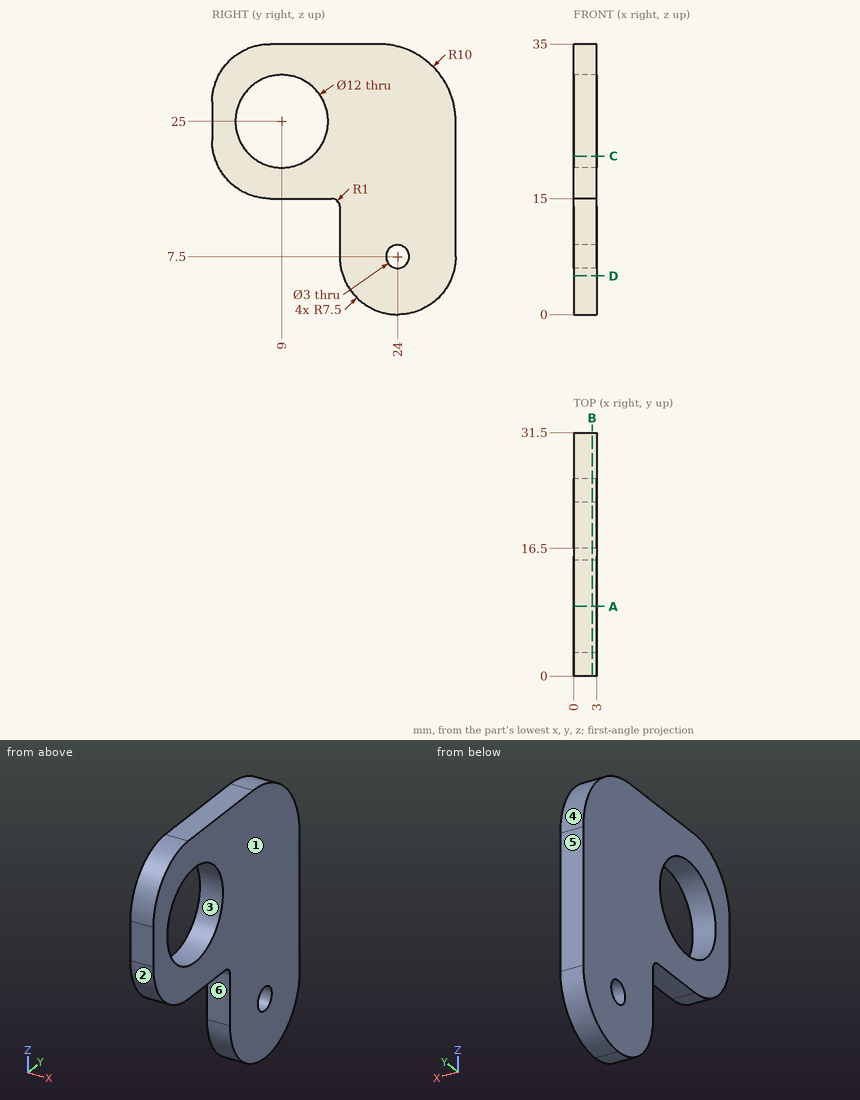
The drawing under review shows one solid part. Ordinate dimensions are in mm from its lowest x, y, z. A direction names the side the tool comes from. Coordinates: 2 decimals unless noted, no trailing zeros. Order: outer loops, then holes, each group sorted by start corner. A loop starts at its lowest first (then second) coordinate and runs counter-clockwise, first axis right, second up. Notation, with made-up numbers: (75, 35) -> (86, 35) arc R21 cw to (86, 50) -> close; hole circle Ø8 at (76.5, 78.25). An arc over 180 degrees is marked (long way). Answer in a Markdown table with one row per item.
(1) Consider section B-B (x = 2.4). State how many separate pieces and enclosed holes the cut face has, plus the area to 3 significant figures.
Answers:
| item | result |
|---|---|
| separate pieces | 1 |
| enclosed holes | 2 |
| area | 665 mm² |
(2) The part is to be moulded in two halves that separate along Z. For the marked faces 1, 2, 3 and 4, say which applies: +Z half, -Z half, draft (parallel to the pull), parting line (faces both ways), or undercut.
Answers:
| item | result |
|---|---|
| face 1 | draft |
| face 2 | -Z half |
| face 3 | undercut |
| face 4 | +Z half |
(3) Consider section C-C (z = 20.5). Write out the cut boundary in (x, y).
Answers:
| item | result |
|---|---|
| outline | (0, 0.27) -> (3, 0.27) -> (3, 5.03) -> (0, 5.03) -> close; (0, 12.97) -> (3, 12.97) -> (3, 31.5) -> (0, 31.5) -> close |
(4) Consider section A-A (y = 9). Write out the cut boundary in (x, z).
Answers:
| item | result |
|---|---|
| outline | (0, 15) -> (3, 15) -> (3, 19) -> (0, 19) -> close; (0, 31) -> (3, 31) -> (3, 35) -> (0, 35) -> close |
(5) Wall thickness on line 1 along Y through (x, z) = (0.9, 7.5); line 2 along Y through (x, z) = (0.5, 14); line 3 along Z through (x, y) = (0.55, 14): over which ranges is each line inside the solid? List them lowest first.
Answers:
| item | result |
|---|---|
| line 1 | 16.5 to 22.5, 25.5 to 31.5 |
| line 2 | 16.5 to 31.5 |
| line 3 | 15 to 21.68, 28.32 to 35 |
(6) Machinability: for the marked faces 5 and 6, which of the approach directions +Z, -Z, +X, -X, +Y, -Y give a long, thin tool a straight path to every point of the face, cutting with its end or side? Answer none if there is none.
Answers:
| item | result |
|---|---|
| face 5 | +Z, -Z, +X, -X, +Y |
| face 6 | -Z, +X, -X, -Y |
(7) Insertion check: pin 1 (11 mm diameter, centred on y = 9, z = 25, fed in from +X); pin 2 (0.9 mm diameter, centred on x = 2, z = 9.5, fed in from -Y). Each pin has a flat end and moves straight along its axis. Give the tip position at first contact, or say it passes through.
Answers:
| item | result |
|---|---|
| pin 1 | through |
| pin 2 | y = 16.5 |
(8) Consider section D-D (z = 5). Write out the cut boundary in (x, y), plus the area to 3 significant figures.
Answers:
| item | result |
|---|---|
| outline | (0, 16.93) -> (3, 16.93) -> (3, 31.07) -> (0, 31.07) -> close |
| area | 42.4 mm² |
